Here's how the part is built. I have some questions about the finished solid (model axes, mm). Coordinates: 2 decimals unless noted, no trailing zeros. Loops run counter-clockwise (first coordinate to the right, second up) from the corner with the lowest first, then second, coordinate; pieces in that order, holes last.
```python
from build123d import *

# Parameters (mm, degrees)
F0_W     = 75
F0_H     = 95
F1_DEPTH = 2
F2_W     = 188
F2_H     = 2
F3_DEPTH = 2
F5_D     = 1.5
F5_DEPTH = 2
F6_W     = 2
F6_H     = 20
F7_DEPTH = 25


with BuildPart() as f1:
    # F0 (on Front) → F1 (new body)
    with BuildSketch(Plane.XZ):
        Polygon((-127.335447, -62.266689), (-6.335447, -62.266689), (-6.335447, 32.733311), (-6.335447, 78.733311), (-127.335447, 78.733311), align=None)
        with Locations((31.164553, -14.766689)):
            Rectangle(F0_W, F0_H)
    extrude(amount=F1_DEPTH)

    # F2 (on face) → F3 (join)
    with BuildSketch(Plane.XZ.offset(2)):
        Polygon((-123.335447, 76.733311), (-125.335447, 76.733311), (-125.335447, -60.266689), (-123.335447, -60.266689), (-123.335447, -58.266689), (-123.335447, 74.733311), align=None)
        Polygon((-8.335447, 76.733311), (-123.335447, 76.733311), (-123.335447, 74.733311), (-10.335447, 74.733311), (-8.335447, 74.733311), align=None)
        with Locations((-29.335447, -59.266689)):
            Rectangle(F2_W, F2_H)
        Polygon((-8.335447, 74.733311), (-10.335447, 74.733311), (-10.335447, 28.733311), (-8.335447, 28.733311), (-8.335447, 30.733311), align=None)
        Polygon((64.664553, -58.266689), (64.664553, -60.266689), (66.664553, -60.266689), (66.664553, 28.733311), (64.664553, 28.733311), align=None)
        Polygon((66.664553, 30.733311), (-8.335447, 30.733311), (-8.335447, 28.733311), (64.664553, 28.733311), (66.664553, 28.733311), align=None)
    extrude(amount=F3_DEPTH)

    # F5
    with Locations(Plane.XZ.offset(2)):
        with Locations((-118.335447, 69.733311), (59.664553, -53.266689)):
            Hole(F5_D / 2, depth=F5_DEPTH)

    # F6 (on face) → F7 (cut)
    with BuildSketch(Plane(origin=(-125.335447, 0, 0), x_dir=(0, -1, 0), z_dir=(-1, 0, 0))):
        with Locations((3, 8.233311)):
            Rectangle(F6_W, F6_H)
    extrude(amount=-F7_DEPTH, mode=Mode.SUBTRACT)


solid = f1.part
```
1. I need wall thicknesses on line 1 along X through (y, z) = (-1.85, 70); line 2 along X through (y, z) = (-2.2, 35); line 3 along Z through (x, y) = (0.5, -2.35). Which ranges of each line are inside material? Lowest first, please.
2. For pin 1 (1 mm diameter, centred on x = 28, y = -1, fed in from +Z); pin 2 (1 mm diameter, centred on x = -8.5, y = -3.5, fed in from +Z); pin 3 (2 mm diameter, centred on y = -1, z = 55.5, fed in from +X), each with a flat end and sliding along its axis, tell me the tip position at first contact or that it passes through.
3. I want a section at A-A (y = -2.9). Please give me the cut outline in (x, z), then the cut area to 3 significant figures.
4. I want a section at C-C (x = -61). Please give me the cut outline in (y, z).
5. I want a section at B-B (z = 62.5). Please give me the cut outline in (x, y).
6. We'd pull the mould along Z, two halves only. Please class faces 1 (the flat face through (-31, 0, 9)), 2 (the flat face through (-31, -2, -6)): +Z half, -Z half, draft (parallel to the pull), parting line (faces both ways), or undercut.
Response values:
1. line 1: x = -127.34 to -119.04, -117.63 to -6.34
1. line 2: x = -125.34 to -123.34, -10.34 to -8.34
1. line 3: z = -60.27 to -58.27, 28.73 to 30.73
2. pin 1: stops at z = 32.73
2. pin 2: stops at z = 76.73
2. pin 3: stops at x = -6.34
3. outline: (-125.34, -60.27) - (66.66, -60.27) - (66.66, 30.73) - (-8.34, 30.73) - (-8.34, 76.73) - (-125.34, 76.73) - (-125.34, 18.23) - (-123.34, 18.23) - (-123.34, 74.73) - (-10.34, 74.73) - (-10.34, 28.73) - (64.66, 28.73) - (64.66, -58.27) - (-123.34, -58.27) - (-123.34, -1.77) - (-125.34, -1.77) - close
3. area: 1,260 mm2
4. outline: (-4, -60.27) - (-2, -60.27) - (-2, -62.27) - (0, -62.27) - (0, 78.73) - (-2, 78.73) - (-2, 76.73) - (-4, 76.73) - (-4, 74.73) - (-2, 74.73) - (-2, -58.27) - (-4, -58.27) - close
5. outline: (-127.34, -2) - (-125.34, -2) - (-125.34, -4) - (-123.34, -4) - (-123.34, -2) - (-10.34, -2) - (-10.34, -4) - (-8.34, -4) - (-8.34, -2) - (-6.34, -2) - (-6.34, 0) - (-127.34, 0) - close
6. face 1: draft
6. face 2: undercut
